Print and shaded views of the part. All mm, measured from the part's lowest x, y and z. A direction names the side the tool comes from. Round coordinates to 2 decimals unless told otherwise and drop trailing zeros. Write each loop counter-clockwise with the first axis right and the second up, starting at its lowest first coordinate (ties: lowest second). Pieces come first, ordered by that corner, then holes. Notation, with made-up numbers: M 14.5,16.5 L 21.5,16.5 A13 cw 21.5,34.5 Z; hole C 74.25,74 d6. An arc over 180 degrees is marked long. Write item = value, one per line.
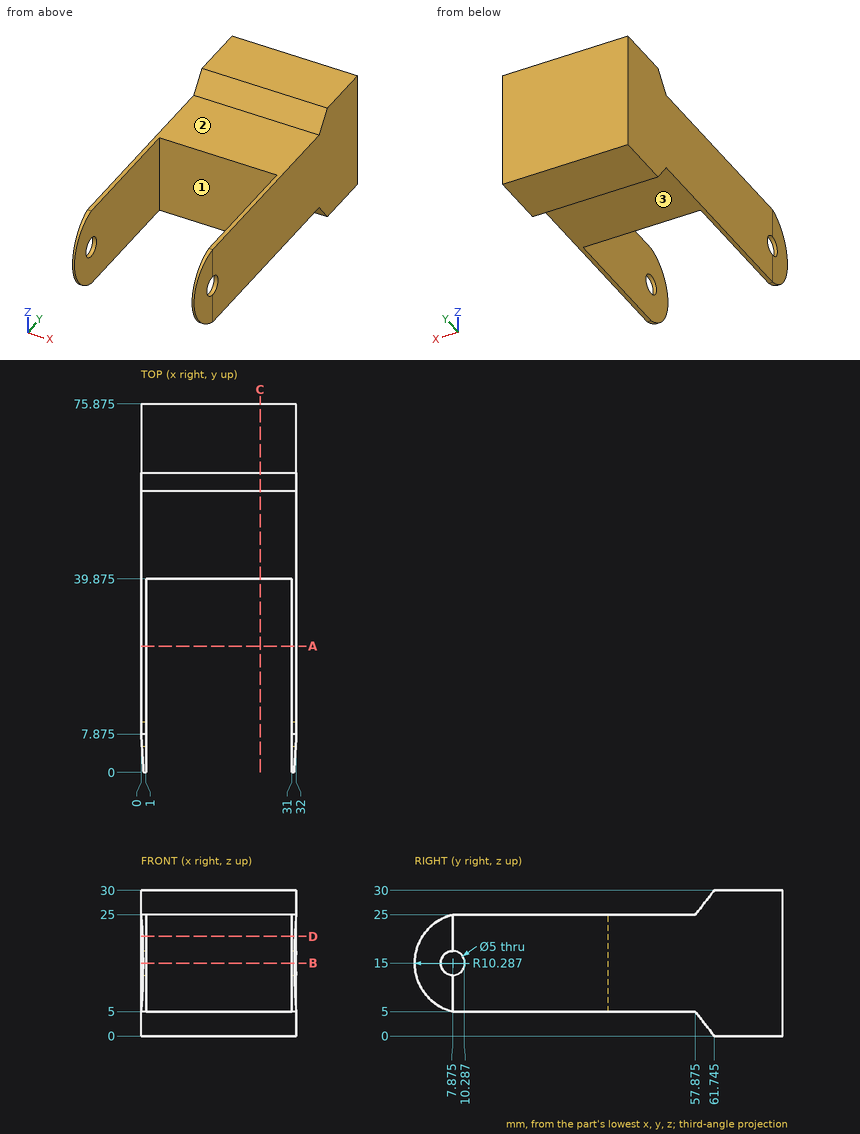
1. Probe probe 1 along X at (y, z) = (11, 24); probe 2 along Y at (x, z) = (31.4, 15) (1 decimal); probe 3 along Y at (x, z) = (14.5, 23.5) (1 decimal). List the from-to ranges inside material, lowest first.
Responses:
probe_1 = 0 to 1, 31 to 32
probe_2 = 0 to 5.4, 10.4 to 75.9
probe_3 = 39.9 to 75.9
2. Band-saw the part on D-D (z = 20.5). List the corners of the cut face in (x, y) (1 decimal).
Responses:
outline = M 0,7.9 L 0.4,1.6 L 1,1.6 L 1,39.9 L 31,39.9 L 31,1.6 L 31.6,1.6 L 32,7.9 L 32,75.9 L 0,75.9 Z
3. Band-saw the part on C-C (x = 24.5). List the corners of the cut face in (y, z) (1 decimal), plus the area to 3 significant figures.
Responses:
outline = M 39.9,5 L 57.9,5 L 61.7,0 L 75.9,0 L 75.9,30 L 61.7,30 L 57.9,25 L 39.9,25 Z
area = 881 mm²
4. Flat gauge pins, fed straight in: pin 1 (1 mm diameter, centred on x = 26.5, z = 7.5, fed in from -Y) (1 decimal); pin 2 (12 mm diameter, centred on x = 6.5, y = 46, fed in from +Z); pin 3 (9.5 mm diameter, centred on x = 10, y = 41, fed in from -Z); pin 4 (4.5 mm diameter, centred on y = 7.87, z = 15, fed in from -X). Where does each tip first touch, or does it go through?
Responses:
pin_1 = 39.9
pin_2 = 25
pin_3 = 5
pin_4 = through
5. Tool access for the marked faces 1, 2 and 3: list every direction of +Z, -Z, +X, -X, +Y, -Y with a clear straight run to the whole face (end or side of a thin tool).
Responses:
face_1 = +Z, -Z, -Y
face_2 = +Z, +X, -X, -Y
face_3 = -Z, +X, -X, -Y
6. Band-saw the part on B-B (z = 15). List the corners of the cut face in (x, y) (1 decimal).
Responses:
outline = M 0,10.4 L 1,10.4 L 1,39.9 L 31,39.9 L 31,10.4 L 32,10.4 L 32,75.9 L 0,75.9 Z; M 0.2,5.4 L 0.5,0 L 1,0 L 1,5.4 Z; M 31,0 L 31.5,0 L 31.8,5.4 L 31,5.4 Z
7. Band-saw the part on A-A (y = 26). List the corners of the cut face in (x, z).
Responses:
outline = M 0,5 L 1,5 L 1,25 L 0,25 Z; M 31,5 L 32,5 L 32,25 L 31,25 Z
